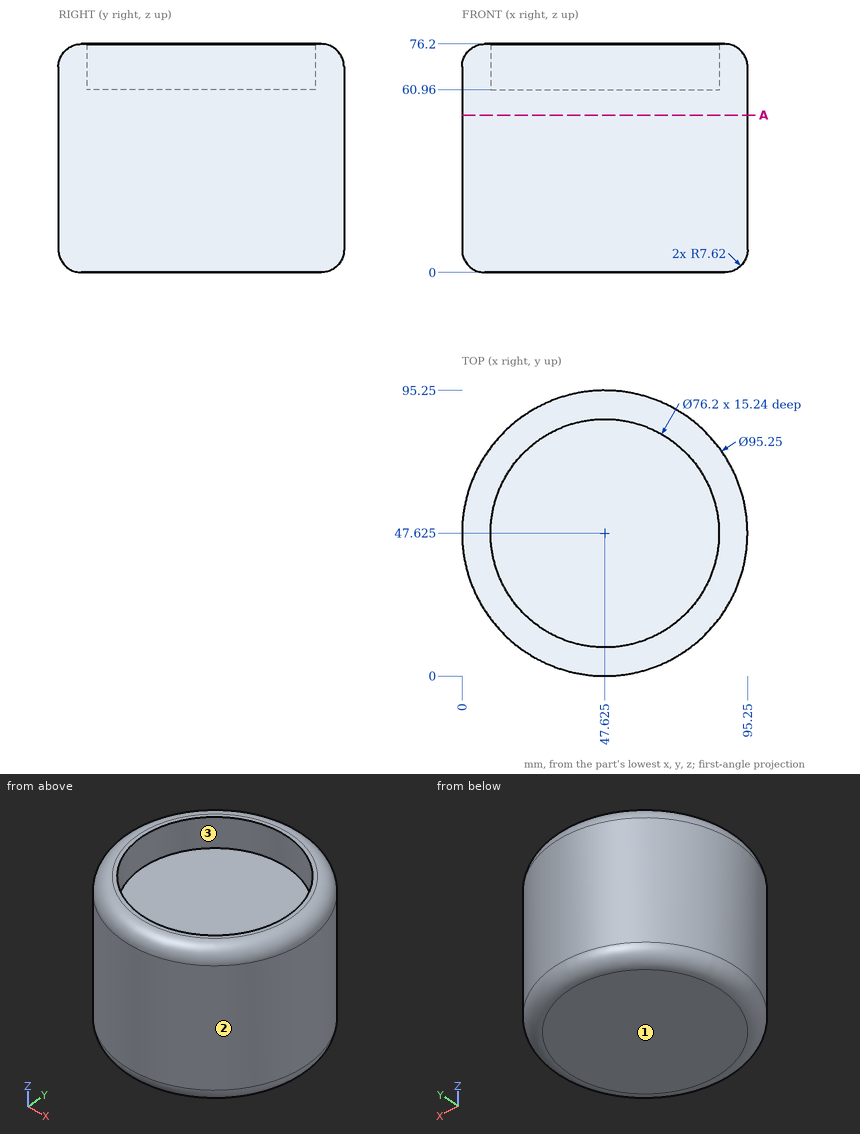
Design review of the part shown in the three views and the two pictorial views. Dimensions are in mm from the part's minimum x, y and z. Give positions to 0.01 mm unless a question says otherwise; leave off trailing zeros. Loops run counter-clockwise (first coordinate to the right, second up) from the corner with the lowest first, then second, coordinate; pieces in that order, holes last. Notation, with made-up numbers: M -13,71 L 44,71 A13 cw 44,87 Z; hole C -29,16.25 d1. An arc over 180 degrees is marked long. Answer as a JSON object with one key per item and string values. Group by question number.
Q1. For probe 1 along Z at (x, y) = (58, 25.5); probe 2 along Y at (x, z) = (28, 63.5); probe 3 along Y at (x, z) = (35, 69), list the stretches that pass through material, from the lowest coordinate up. Write a range as [from, to].
Q2. Mouldability with a two-part tool opening along Y and no side actions: class the marked faces 1, 2 and 3 as +Y half, -Y half, draft (parallel to the pull), parting line (faces both ways), or undercut.
Q3. Insertion check: P1, Ø8, axis at y = 12, z = 42.5, coming from the -X side; P2, Ø5, axis at x = 82.5, y = 34.5, coming from the +Z side; P3, Ø8, axis at x = 57.5, z = 13.5, coming from the +Y side; P4, Ø4, axis at x = 14.5, y = 60, coming from the +Z side. Each pin has a flat end and moves straight along its axis. Give the tip position at first contact, or say it passes through.
Q4. Add section A-A on z = 52.5. Give the boundary of the cut face in (x, y) (3 decimals), and give its area (3 significant figures).
Checked values:
{
 "1": {"probe 1": "[0, 60.96]", "probe 2": "[4.23, 14.97], [80.28, 91.02]", "probe 3": "[1.72, 11.68], [83.57, 93.53]"},
 "2": {"face 1": "draft", "face 2": "parting line", "face 3": "undercut"},
 "3": {"P1": "x = 12.02", "P2": "z = 76.2", "P3": "y = 94.89", "P4": "z = 60.96"},
 "4": {"outline": "C 47.625,47.625 d95.25", "area": "7,130 mm²"}
}
